For this review, take the finished solid that the model builds, in its own axes (mm). Coordinates: 2 decimals unless noted, no trailing zeros. Order: outer loops, then holes, each group sorted by start corner. A loop starts at its lowest first (then second) coordinate and runs counter-clockwise, first axis right, second up.
from build123d import *

# Parameters (mm, degrees)
BASE_EXTRUDE_DEPTH = 63.5
FILLET1_R          = 38.1


with BuildPart() as part:
    # Sketch7 → Base-Extrude (new, symmetric)
    with BuildSketch(Plane(origin=(114.3, 0, 0), x_dir=(0, 0, -1), z_dir=(1, 0, 0))):
        with BuildLine():
            ThreePointArc((37.885471858, -742.213802936), (-33.838948323, -692.9538134), (-87.396251362, -761.528986099))
            ThreePointArc((-87.396251362, -761.528986099), (-58.651901192, -967.339401786), (-10.701792985, -1169.539678727))
            ThreePointArc((-10.701792985, -1169.539678727), (31.347433103, -1196.725838045), (64.014969584, -1158.777758602))
            ThreePointArc((64.014969584, -1158.777758602), (64.297743258, -1113.02154154), (65.715717531, -1067.286426914))
            ThreePointArc((65.715717531, -1067.286426914), (62.282866841, -903.852702509), (37.885471858, -742.213802936))
        make_face()
    extrude(amount=BASE_EXTRUDE_DEPTH, both=True)

    # Fillet1
    fillet1_edges = [part.edges().sort_by_distance(p)[0] for p in [
        (50.8, -903.852702509, -62.282866841),
        (177.8, -903.852702509, -62.282866841),
        (50.8, -1113.02154154, -64.297743258),
        (177.8, -1113.02154154, -64.297743258),
        (50.8, -1196.725838045, -31.347433103),
        (177.8, -1196.725838045, -31.347433103),
        (50.8, -967.339401786, 58.651901192),
        (177.8, -967.339401786, 58.651901192),
        (177.8, -692.9538134, 33.838948323),
        (50.8, -692.9538134, 33.838948323),
    ]]
    fillet(fillet1_edges, radius=FILLET1_R)


solid = part.part
1. To check wall thickness, follow L1, parallel to X at y = -745, z = -1; L2, parallel to Z at x = 58.5, y = -948.5; L3, parallel to Z at x = 154, y = -1118. State the ranges of each line that lie inside material, in increasing order.
Answer below:
L1: x = 50.85 to 177.75
L2: z = -50.16 to 46.73
L3: z = -61.43 to 21.96
2. Take a section at A-A, the plane x = 116. Give the boundary of the cut face in (y, z), plus the area to 3 significant figures.
Answer below:
outline: (-1169.54, 10.7) arc R38.1 ccw to (-1158.78, -64.01) arc R1844.04 cw to (-1067.29, -65.72) arc R1270 ccw to (-742.21, -37.89) arc R63.5 ccw to (-761.53, 87.4) arc R2209.8 ccw to start
area: 56,200 mm2
3. Clearance check with flat-ended pins moving along their axes: pin 1 Ø8 at (x, y) = (128.5, -763.5) entering from +Z; pin 2 Ø4 at (x, z) = (77.5, -35.5) entering from -Y; pin 3 Ø12 at (x, z) = (76.5, -16) entering from -Y. State where each tip first meets the part, or that it passes through.
Answer below:
pin 1: stops at z = 87.55
pin 2: stops at y = -1194.87
pin 3: stops at y = -1195.81
